Solid Edge part; units mm, degrees
sketch "Sketch1" plane through (0, 0, 0) normal (0, -1, 0) x (1, 0, 0)
  line L0 (12.5, 0) -> (12.5, 11)
  line L1 (12.5, 11) -> (10, 11)
  line L2 (10, 11) -> (10, 3.5)
  line L3 (10, 3.5) -> (2.5, 3.5)
  line L4 (2.5, 3.5) -> (2.5, 11)
  line L5 (2.5, 11) -> (0, 11)
  line L6 (0, 11) -> (0, 0)
  line L7 (0, 0) -> (12.5, 0)
extrude "Protrusion1" add sketch "Sketch1" against normal blind 144
sketch "Sketch2" plane through (6.25, 0, 5.5) normal (0, -1, 0) x (1, 0, 0)
  line L0 (-3.75, 5.5) -> (3.75, 5.5)
  line L1 (3.75, 5.5) -> (3.75, -2)
  line L2 (3.75, -2) -> (-3.75, -2)
  line L3 (-3.75, -2) -> (-3.75, 5.5)
extrude "ExtrudedProtrusion_2" add sketch "Sketch2" against normal blind 2.5
sketch "Sketch3" plane through (6.25, 77.25, 3.5) normal (0, 0, 1) x (0, 1, 0)
  circle A0 centre (-68.25, 0) radius 1.65
  circle A1 centre (-9.25, 0) radius 1.65
  circle A2 centre (61.75, 0) radius 1.65
extrude "Cutout1" cut sketch "Sketch3" against normal through all
chamfer "Countersink" distance 1.67 angle 45 3 edges at (6.25, 66.35, 3.5) (6.25, 7.35, 3.5) (6.25, 137.35, 3.5)
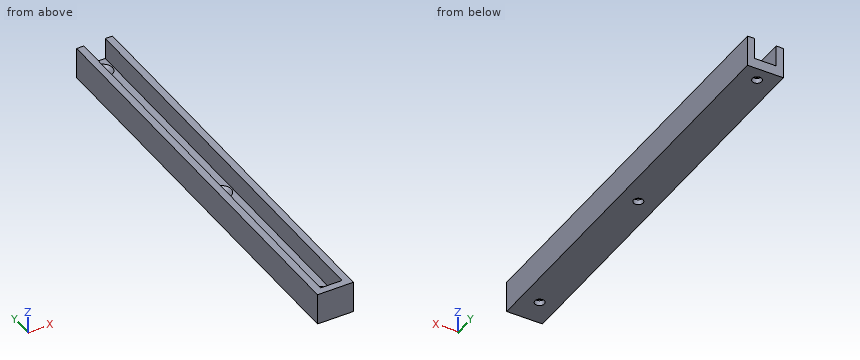
Build history of the part. All positions in model axes, mm. Round coordinates to 2 decimals unless told otherwise and drop trailing zeros. Write each loop counter-clockwise with the first axis right and the second up, starting at its lowest first coordinate (ties: lowest second). Pieces come first, ordered by that corner, then holes. Notation, with made-up numbers: (-4.75, 8) - (28.25, 8) arc R36 ccw to (28.25, 44) - close; hole circle Ø6 at (-27, 29.5). An arc over 180 degrees is marked (long way). Answer as CSV lines item,"result".
Q1. Cut at C-C (z = 5.5). Write the cut outline in (x, y), and give its area (3 significant figures).
Report:
outline,"(0, 0) - (12.5, 0) - (12.5, 144) - (10, 144) - (10, 2.5) - (2.5, 2.5) - (2.5, 144) - (0, 144) - close"
area,"739 mm^2"
Q2. Cut at D-D (y = 100). Write the cut outline in (x, z), and give its area (4 significant figures).
Report:
outline,"(0, 0) - (12.5, 0) - (12.5, 11) - (10, 11) - (10, 3.5) - (2.5, 3.5) - (2.5, 11) - (0, 11) - close"
area,"81.25 mm^2"
Q3. Drill centre lines: probe 1 along Y at (x, z) = (6.25, 0.6); probe 2 along X at (y, z) = (75, 9.75); probe 3 along X at (y, z) = (68, 0.6). Where is each one in solid material? Low to high. Write a range as [from, to].
Report:
probe 1,"y = [0, 7.35], [10.65, 66.35], [69.65, 137.35], [140.65, 144]"
probe 2,"x = [0, 2.5], [10, 12.5]"
probe 3,"x = [0, 4.6], [7.9, 12.5]"
Q4. Cut at A-A (y = 139). Write the cut outline in (x, z), and give its area (3 significant figures).
Report:
outline,"(0, 0) - (4.6, 0) - (4.6, 1.83) - (2.93, 3.5) - (2.5, 3.5) - (2.5, 11) - (0, 11) - close; (7.9, 0) - (12.5, 0) - (12.5, 11) - (10, 11) - (10, 3.5) - (9.57, 3.5) - (7.9, 1.83) - close"
area,"66.9 mm^2"
Q5. Cut at B-B (x = 6.25). Write the cut outline in (y, z), and give its area (3 significant figures).
Report:
outline,"(0, 0) - (7.35, 0) - (7.35, 1.83) - (5.68, 3.5) - (2.5, 3.5) - (2.5, 11) - (0, 11) - close; (10.65, 0) - (66.35, 0) - (66.35, 1.83) - (64.68, 3.5) - (12.32, 3.5) - (10.65, 1.83) - close; (69.65, 0) - (137.35, 0) - (137.35, 1.83) - (135.68, 3.5) - (71.32, 3.5) - (69.65, 1.83) - close; (140.65, 0) - (144, 0) - (144, 3.5) - (142.32, 3.5) - (140.65, 1.83) - close"
area,"480 mm^2"
Q6. Drop flat-ended pins along their axis: pin 1 (3 mm diameter, centred on x = 6.25, y = 139, fed in from +Z); pin 2 (6 mm diameter, centred on x = 6, y = 86.5, fed in from +Z). Give the stop position or say it passes through.
Report:
pin 1,"passes through"
pin 2,"stops at z = 3.5"
